Can you work these out from the drawing? Everything is in mm from the part's minimum corner. A direction names the side the tool comes from. Round coordinates to 2 decimals unless told otherwise and drop trailing zeros. Loops run counter-clockwise (first coordinate to the right, second up) from the corner with the lowest first, then second, coordinate; pieces in that order, holes last. Notation, with made-up numbers: (76.5, 75) -> (101.5, 75) arc R20 ccw to (101.5, 82) -> close; hole circle Ø3 at (17.5, -31.5). An arc over 180 degrees is marked (long way). One line per item, written item: value.
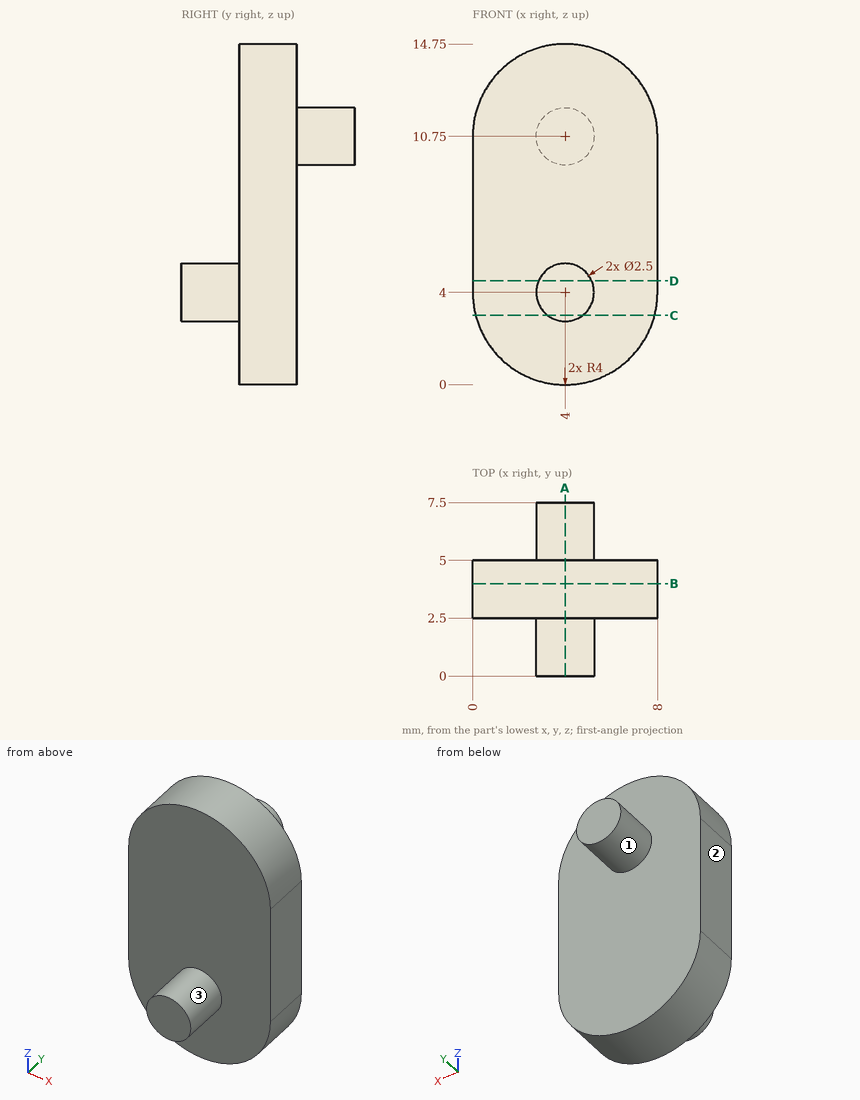
(1) For pin 1 Ø2 at (y, z) = (1, 3) entering from -X; pin 2 Ø2 at (y, z) = (2.5, 2.5) entering from -X; pin 3 Ø2.5 at (x, z) = (6, 7) entering from +Y, each with a flat end and sliding along its axis, tell me the tip position at first contact or that it passes through.
Results below:
pin 1: stops at x = 2.75
pin 2: stops at x = 0.03
pin 3: stops at y = 5
(2) Imagine slicing it at D-D on z = 4.5. Write out the boundary of the cut face in (x, y), then the cut area to 3 significant figures.
Results below:
outline: (0, 2.5) -> (2.85, 2.5) -> (2.85, 0) -> (5.15, 0) -> (5.15, 2.5) -> (8, 2.5) -> (8, 5) -> (0, 5) -> close
area: 25.7 mm²
(3) Please list where these lines run through material, in increasing order: L1, parallel to Y at x = 3.25, z = 9; L2, parallel to Y at x = 3.5, z = 4.75; L3, parallel to Z at x = 6.25, y = 4.25.
Results below:
L1: y = 2.5 to 5
L2: y = 0 to 5
L3: z = 0.69 to 14.06
(4) Imagine slicing it at C-C on z = 3. Write out the boundary of the cut face in (x, y).
Results below:
outline: (0.13, 2.5) -> (3.25, 2.5) -> (3.25, 0) -> (4.75, 0) -> (4.75, 2.5) -> (7.87, 2.5) -> (7.87, 5) -> (0.13, 5) -> close
(5) Imagine slicing it at B-B on y = 4. Write out the boundary of the cut face in (x, z), then the cut area to 3 significant figures.
Results below:
outline: (0, 4) arc R4 ccw to (8, 4) -> (8, 10.75) arc R4 ccw to (0, 10.75) -> close
area: 104 mm²
(6) Imagine slicing it at A-A on x = 4. Write out the boundary of the cut face in (y, z), then the cut area to 3 significant figures.
Results below:
outline: (0, 2.75) -> (2.5, 2.75) -> (2.5, 0) -> (5, 0) -> (5, 9.5) -> (7.5, 9.5) -> (7.5, 12) -> (5, 12) -> (5, 14.75) -> (2.5, 14.75) -> (2.5, 5.25) -> (0, 5.25) -> close
area: 49.4 mm²
(7) On a 3-axis mill with a long thin cutter (end or side, diameter ignored), from which of +Z, -Z, +X, -X, +Y, -Y can I reach the whole of each face in a straight line? I mean the marked faces 1, 2 and 3. Say none if no direction works.
Results below:
face 1: +Y
face 2: +Z, -Z, -X, +Y, -Y
face 3: -Y
